Part model, mm, in its own coordinate system. Face numbers are marked on the shaded views. A direction names the side the tool comes from. Give positions to 0.01 mm unless a question says otherwise; leave off trailing zeros. Write each loop counter-clockwise with the first axis right and the second up, starting at its lowest first coordinate (ties: lowest second). Pieces come first, ordered by that corner, then holes.
from build123d import *

# Parameters (mm, degrees)
F1_DEPTH = 89
F2_R     = 5
F3_T     = -2.5


with BuildPart() as f1:
    # F0 (on Top) → F1 (new body)
    with BuildSketch(Plane.XY):
        Polygon((-21.937249, 72.949414), (-34.437249, -16.178304), (20.562751, -16.178304), (8.062751, 72.949414), align=None)
    extrude(amount=F1_DEPTH)

    # F2
    f2_edges = [f1.edges().sort_by_distance(p)[0] for p in [
        (-34.437249, -16.178304, 44.5),
        (20.562751, -16.178304, 44.5),
        (8.062751, 72.949414, 44.5),
        (-21.937249, 72.949414, 44.5),
    ]]
    fillet(f2_edges, radius=F2_R)

    # F3
    f3_openings = [f1.faces().sort_by_distance(p)[0] for p in [
        (-6.937249, 24.070878, 89),
    ]]
    offset(amount=F3_T, openings=f3_openings)


solid = f1.part
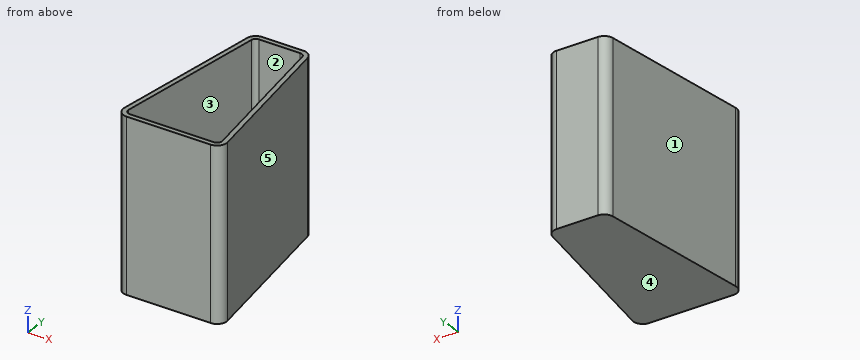
1) Flat gauge pins, fed straight in: P1, Ø8, axis at x = -14, y = 53.5, coming from the +Z side; P2, Ø4, axis at y = 47, z = 72, coming from the +X side; P3, Ø4, axis at y = 55.5, z = 55, coming from the +X side. Where does each tip first touch, or does it go through?
Check result:
P1: stops at z = 2.5
P2: stops at x = 11.98
P3: stops at x = 10.79
2) Mould opens along Y. For the marked faces 3, 4 and 5 say: +Y half, -Y half, draft (parallel to the pull), parting line (faces both ways), or undercut.
Check result:
face 3: undercut
face 4: draft
face 5: +Y half
3) Drill centre lines: L1, parallel to Y at x = -17, z = 83.5; L2, parallel to X at y = 7, z = 67; L3, parallel to Z at x = -12, y = -9. Where is each one in solid material? Low to high.
Check result:
L1: y = -16.18 to -13.68, 70.45 to 72.95
L2: x = -31.19 to -28.66, 14.79 to 17.31
L3: z = 0 to 2.5
4) Saw through at C-C (x = -6). Write the cut outline in (y, z), and give its area (3 significant figures).
Check result:
outline: (-16.18, 0) - (72.95, 0) - (72.95, 89) - (70.45, 89) - (70.45, 2.5) - (-13.68, 2.5) - (-13.68, 89) - (-16.18, 89) - close
area: 655 mm2
5) Saw through at B-B (y = 9.5). Write the cut outline in (x, z), and give its area (3 significant figures).
Check result:
outline: (-30.84, 0) - (16.96, 0) - (16.96, 89) - (14.44, 89) - (14.44, 2.5) - (-28.31, 2.5) - (-28.31, 89) - (-30.84, 89) - close
area: 556 mm2
6) 3-axis set-ups, long thin cutter, end or side, ignore diameter. For the marked faces 1 and 2: which of +Z, -Z, +X, -X, +Y, -Y reach the whole face in a straight line?
Check result:
face 1: +Z, -Z, -X, +Y
face 2: +Z
7) Saw through at A-A (z = 23). Write the cut outline in (x, y).
Check result:
outline: (-33.64, -10.48) arc R5 ccw to (-28.69, -16.18) - (14.81, -16.18) arc R5 ccw to (19.76, -10.48) - (8.67, 68.64) arc R5 ccw to (3.72, 72.95) - (-17.59, 72.95) arc R5 ccw to (-22.54, 68.64) - close; hole (-31.16, -10.83) arc R2.5 ccw to (-28.69, -13.68) - (14.81, -13.68) arc R2.5 ccw to (17.29, -10.83) - (6.19, 68.3) arc R2.5 ccw to (3.72, 70.45) - (-17.59, 70.45) arc R2.5 ccw to (-20.07, 68.3) - close
